Build history of the part. All positions in model axes, mm. Round coordinates to 2 decimals unless told otherwise and drop trailing zeros. Loops run counter-clockwise (first coordinate to the right, second up) from the corner with the lowest first, then second, coordinate; pieces in that order, holes last. Notation, with made-up numbers: (64, 4.5) - (80, 4.5) arc R24 cw to (80, 26.5) - close; hole circle Ø1 at (-7, -27). An arc over 180 degrees is marked (long way). Put each result on its own line as item: value. Start each with the question number.
from build123d import *

# Parameters (mm, degrees)
SKETCH1_W           = 30
SKETCH1_H           = 5
SKETCH1_R           = 1
BOSS_EXTRUDE1_DEPTH = 2
FILLET1_R           = 2.5


with BuildPart() as part:
    # Sketch1 → Boss-Extrude1 (new body)
    with BuildSketch(Plane.XY):
        Rectangle(SKETCH1_W, SKETCH1_H)
        with Locations((12.646126356, 0)):
            Circle(SKETCH1_R, mode=Mode.SUBTRACT)
        with Locations(Location((-12.646126356, 0, 0), (0, 0, 180))):
            Circle(SKETCH1_R, mode=Mode.SUBTRACT)
    extrude(amount=BOSS_EXTRUDE1_DEPTH)

    # Fillet1
    fillet1_edges = [part.edges().sort_by_distance(p)[0] for p in [
        (-15, -2.5, 1),
        (-15, 2.5, 1),
        (15, -2.5, 1),
        (15, 2.5, 1),
    ]]
    fillet(fillet1_edges, radius=FILLET1_R - 0.0001)  # a hair under: the kernel refuses the full size


solid = part.part
Item 1: Slice it at A-A (z = 0.5). Give the number of separate pieces and of enclosed holes in the cut face, plus the area to 3 significant figures.
Item 2: Drop flat-ended pins along their axis: pin 1 Ø1.6 at (x, y) = (12.65, 0) entering from -Z; pin 2 Ø3 at (x, y) = (-12.65, 0) entering from -Z. Give the stop position or say it passes through.
Item 3: Two-plate mould, pull along X, no slides. Class faces 1 (the cylindrical face through (-14, 2, 1)), 2 (the flat face through (0, 0, 2)), 3 (the cylindrical face through (14, 2, 1)), 4 (the cylindrical face through (-11.647, -0.044, 0.986)): pulls with the +X half, pulls with the -X half, needs draft (parallel to the pull), parting line crosses it, or undercut.
Item 4: Slice it at B-B (y = -0.7). Give the cut face in (x, z).
Item 5: Drill centre lines: probe 1 along X at (y, z) = (-0.8, 1.2); probe 2 along X at (y, z) = (0.85, 1.6); probe 3 along Y at (x, z) = (13, 0.7). Where is each one in solid material? Low to high. Write a range as [from, to].
Item 6: Slice it at C-C (y = 1.85). Give the cut face in (x, z).
Computed values:
1. separate pieces: 1
1. enclosed holes: 2
1. area: 138 mm^2
2. pin 1: passes through
2. pin 2: stops at z = 0
3. face 1: pulls with the -X half
3. face 2: needs draft
3. face 3: pulls with the +X half
3. face 4: undercut
4. outline: (-14.9, 0) - (-13.36, 0) - (-13.36, 2) - (-14.9, 2) - close; (-11.93, 0) - (11.93, 0) - (11.93, 2) - (-11.93, 2) - close; (13.36, 0) - (14.9, 0) - (14.9, 2) - (13.36, 2) - close
5. probe 1: x = [-14.87, -13.25], [-12.05, 12.05], [13.25, 14.87]
5. probe 2: x = [-14.85, -13.17], [-12.12, 12.12], [13.17, 14.85]
5. probe 3: y = [-2.45, -0.94], [0.94, 2.45]
6. outline: (-14.18, 0) - (14.18, 0) - (14.18, 2) - (-14.18, 2) - close
